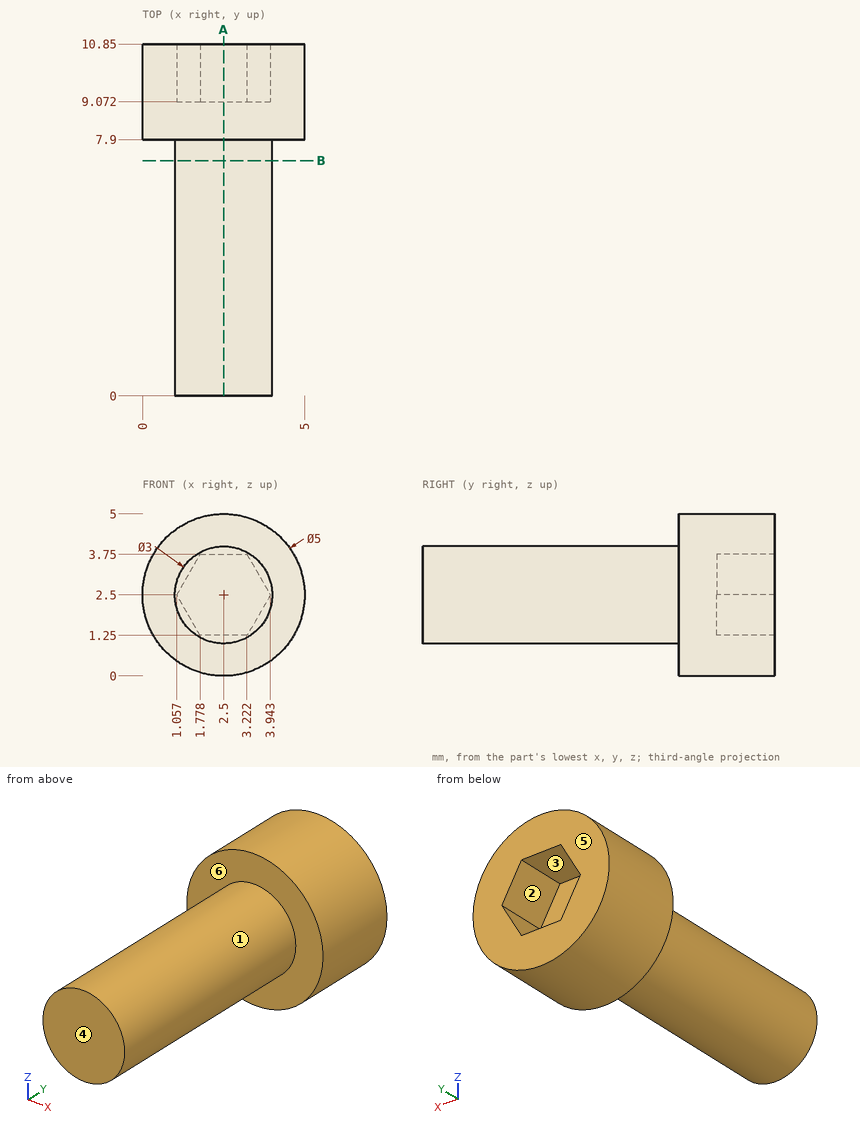
Study the drawing (mm; zero at the part's minimum x, y, z) and answer. A direction names the side the tool comes from. Coordinates: 2 decimals unless noted, no trailing zeros. Write each loop counter-clockwise with the first axis right and the second up, starting at its lowest first coordinate (ties: lowest second). Pieces come first, ordered by that corner, then holes. Notation, with made-up numbers: (18.25, -4) - (45.25, -4) arc R20 ccw to (45.25, 8) - close; hole circle Ø5 at (-1, 32.25). An arc over 180 degrees is marked (long way). One line per item, written item: value.
1) A tool of negligible diameter and unlimited length cuts with its end or side. For the marked faces 5 and 6, from which of +Z, -Z, +X, -X, +Y, -Y can it reach the whole face along a straight path? Write none if from no direction.
Geometry check:
face 5: +Z, -Z, +X, -X, +Y
face 6: -Y
2) For a pull along Z with two mould halves and no side action, classify the marked faces 1, 2, 3 and 4 as pulls with the +Z half, pulls with the -Z half, needs draft (parallel to the pull), parting line crosses it, or undercut.
Geometry check:
face 1: parting line crosses it
face 2: undercut
face 3: undercut
face 4: needs draft
3) Each of these flat-tipped pins is pushed along its axis until it touches: pin 1 Ø1.5 at (y, z) = (4, 2) entering from +X; pin 2 Ø2 at (x, z) = (1, 1) entering from -Y; pin 3 Ø1.5 at (y, z) = (9, 4.5) entering from +X (1 decimal). Where does it stop, or does it pass through?
Geometry check:
pin 1: stops at x = 4
pin 2: stops at y = 0
pin 3: stops at x = 4.7
4) Find section B-B (y = 7.25). Give the vertices of the cut face in (x, z).
Geometry check:
outline: circle Ø3 at (2.5, 2.5)
5) Find section A-A (x = 2.5). Give the vertices of the cut face in (y, z), and give its area (3 significant figures).
Geometry check:
outline: (0, 1) - (7.9, 1) - (7.9, 0) - (10.85, 0) - (10.85, 1.25) - (9.07, 1.25) - (9.07, 3.75) - (10.85, 3.75) - (10.85, 5) - (7.9, 5) - (7.9, 4) - (0, 4) - close
area: 34.0 mm2
6) Consider line 1 along Y through (x, z) = (1.35, 2.4); line 2 along Z through (x, y) = (2.1, 5.5) (1 decimal); line 3 along Z through (x, y) = (2.5, 3.25). Determine where each line is inside the solid, lowest interval first. Write a range as from..to.
Geometry check:
line 1: y = 0..9.07
line 2: z = 1.1..3.9
line 3: z = 1..4
